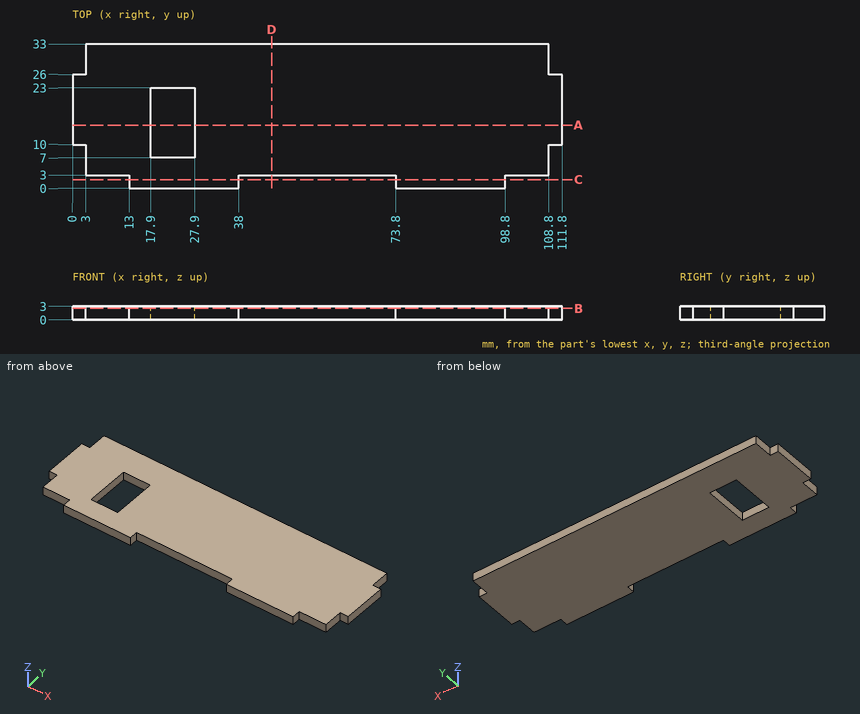
Design review of the part shown in the three views and the two pictorial views. Dimensions are in mm from the part's minimum x, y and z. Round coordinates to 2 decimals unless told otherwise and drop trailing zeros. Loops run counter-clockwise (first coordinate to the right, second up) from the corner with the lowest first, then second, coordinate; pieces in that order, holes last.
1) Consider section D-D on x = 45.5. State the section outline as (y, z) points, then the cut area to 3 significant figures.
Values follow:
outline: (3, 0) - (33, 0) - (33, 3) - (3, 3) - close
area: 90.0 mm2
2) Consider section C-C on y = 2. State the section outline as (x, z) points, then the cut area to 3 significant figures.
Values follow:
outline: (13, 0) - (38, 0) - (38, 3) - (13, 3) - close; (73.8, 0) - (98.8, 0) - (98.8, 3) - (73.8, 3) - close
area: 150 mm2
3) Consider section A-A on y = 14.5. State the section outline as (x, z) points.
Values follow:
outline: (0, 0) - (17.9, 0) - (17.9, 3) - (0, 3) - close; (27.9, 0) - (111.8, 0) - (111.8, 3) - (27.9, 3) - close
4) Wall thickness on line 1 along Y through (x, z) = (20, 2.05); line 2 along X through (y, z) = (16.5, 2.05); line 3 along X through (y, z) = (9, 2.45): over which ranges is each line inside the solid? List them lowest first.
Values follow:
line 1: y = 0 to 7, 23 to 33
line 2: x = 0 to 17.9, 27.9 to 111.8
line 3: x = 3 to 17.9, 27.9 to 108.8
5) Consider section B-B on z = 2.55. State the section outline as (x, y) points.
Values follow:
outline: (0, 10) - (3, 10) - (3, 3) - (13, 3) - (13, 0) - (38, 0) - (38, 3) - (73.8, 3) - (73.8, 0) - (98.8, 0) - (98.8, 3) - (108.8, 3) - (108.8, 10) - (111.8, 10) - (111.8, 26) - (108.8, 26) - (108.8, 33) - (3, 33) - (3, 26) - (0, 26) - close; hole (17.9, 7) - (27.9, 7) - (27.9, 23) - (17.9, 23) - close
6) Clearance check with flat-ended pins moving along their axes: P1, Ø1.5, axis at y = 1, z = 1, coming from the +X side; P2, Ø0.9, axis at x = 2, z = 2, coming from the +Y side; P3, Ø1.5, axis at x = 1, z = 1.5, coming from the -Y side. State where each tip first meets the part, or that it passes through.
Values follow:
P1: stops at x = 98.8
P2: stops at y = 26
P3: stops at y = 10
